Check sheet for the modelled part. Datum: model origin and axes. Units: mm. Face numbers are marked on the shaded views. A direction names the side the tool comes from. Give positions to 0.01 mm unless a question says otherwise; leave off trailing zeros. Order: outer loops, then holes, each group sorted by start corner. A loop starts at its lowest first (then second) coordinate and runs counter-clockwise, first axis right, second up.
```python
from build123d import *

# Parameters (mm, degrees)
F0_R     = 1.6
F1_DEPTH = 3.5
F3_COUNT = 16
F5_R     = 6.5
F6_DEPTH = 1
F7_R     = 6.5
F8_DEPTH = 1
F9_DEPTH = 12.5


with BuildPart() as f1:
    # F0 (on Top) → F1 (new body, symmetric)
    with BuildSketch(Plane.XY):
        with BuildLine():
            ThreePointArc((-0.6307960914, 4.7079290873), (-3.1277962342, -3.5748273689), (4.75, 0))
            ThreePointArc((4.75, 0), (3.5748273689, 3.1277962342), (0.6307960914, 4.7079290873))
            Line((0.6307960914, 4.7079290873), (0.75, 4.3804190402))
            Line((0.75, 4.3804190402), (-0.75, 4.3804190402))
            Line((-0.75, 4.3804190402), (-0.6307960914, 4.7079290873))
        make_face()
        Circle(F0_R, mode=Mode.SUBTRACT)
        with BuildLine():
            ThreePointArc((-0.6307960914, 4.7079290873), (0, 4.75), (0.6307960914, 4.7079290873))
            Line((0.6307960914, 4.7079290873), (0.3607043675, 5.45))
            Line((0.3607043675, 5.45), (-0.3607043675, 5.45))
            Line((-0.3607043675, 5.45), (-0.6307960914, 4.7079290873))
        make_face()
        with BuildLine():
            Line((0.75, 4.3804190402), (0.6307960914, 4.7079290873))
            ThreePointArc((0.6307960914, 4.7079290873), (0, 4.75), (-0.6307960914, 4.7079290873))
            Line((-0.6307960914, 4.7079290873), (-0.75, 4.3804190402))
            Line((-0.75, 4.3804190402), (0.75, 4.3804190402))
        make_face()
    extrude(amount=F1_DEPTH, both=True)


with BuildPart() as f3_1:
    # F3: instance of F1
    add(f1.part.rotate(Axis((0, 0, 0.113066053), (0, 0, -1)), 1 * 360 / F3_COUNT))


with BuildPart() as f3_2:
    # F3: instance of F1
    add(f1.part.rotate(Axis((0, 0, 0.113066053), (0, 0, -1)), 2 * 360 / F3_COUNT))


with BuildPart() as f3_3:
    # F3: instance of F1
    add(f1.part.rotate(Axis((0, 0, 0.113066053), (0, 0, -1)), 3 * 360 / F3_COUNT))


with BuildPart() as f3_4:
    # F3: instance of F1
    add(f1.part.rotate(Axis((0, 0, 0.113066053), (0, 0, -1)), 4 * 360 / F3_COUNT))


with BuildPart() as f3_5:
    # F3: instance of F1
    add(f1.part.rotate(Axis((0, 0, 0.113066053), (0, 0, -1)), 5 * 360 / F3_COUNT))


with BuildPart() as f3_6:
    # F3: instance of F1
    add(f1.part.rotate(Axis((0, 0, 0.113066053), (0, 0, -1)), 6 * 360 / F3_COUNT))


with BuildPart() as f3_7:
    # F3: instance of F1
    add(f1.part.rotate(Axis((0, 0, 0.113066053), (0, 0, -1)), 7 * 360 / F3_COUNT))


with BuildPart() as f3_8:
    # F3: instance of F1
    add(f1.part.rotate(Axis((0, 0, 0.113066053), (0, 0, -1)), 8 * 360 / F3_COUNT))


with BuildPart() as f3_9:
    # F3: instance of F1
    add(f1.part.rotate(Axis((0, 0, 0.113066053), (0, 0, -1)), 9 * 360 / F3_COUNT))


with BuildPart() as f3_10:
    # F3: instance of F1
    add(f1.part.rotate(Axis((0, 0, 0.113066053), (0, 0, -1)), 10 * 360 / F3_COUNT))


with BuildPart() as f3_11:
    # F3: instance of F1
    add(f1.part.rotate(Axis((0, 0, 0.113066053), (0, 0, -1)), 11 * 360 / F3_COUNT))


with BuildPart() as f3_12:
    # F3: instance of F1
    add(f1.part.rotate(Axis((0, 0, 0.113066053), (0, 0, -1)), 12 * 360 / F3_COUNT))


with BuildPart() as f3_13:
    # F3: instance of F1
    add(f1.part.rotate(Axis((0, 0, 0.113066053), (0, 0, -1)), 13 * 360 / F3_COUNT))


with BuildPart() as f3_14:
    # F3: instance of F1
    add(f1.part.rotate(Axis((0, 0, 0.113066053), (0, 0, -1)), 14 * 360 / F3_COUNT))


with BuildPart() as f3_15:
    # F3: instance of F1
    add(f1.part.rotate(Axis((0, 0, 0.113066053), (0, 0, -1)), 15 * 360 / F3_COUNT))


with BuildPart() as f3_1_1:
    add(f3_1.part)

    # F4: union F3_2, F3_3, F3_4, F3_5, F3_7, F3_9, F3_10, F3_8, F3_6, F3_11, F3_12, F3_14, F1, F3_13, F3_15
    add(f3_2.part)
    add(f3_3.part)
    add(f3_4.part)
    add(f3_5.part)
    add(f3_7.part)
    add(f3_9.part)
    add(f3_10.part)
    add(f3_8.part)
    add(f3_6.part)
    add(f3_11.part)
    add(f3_12.part)
    add(f3_14.part)
    add(f1.part)
    add(f3_13.part)
    add(f3_15.part)

    # F5 (on face) → F6 (join)
    with BuildSketch(Plane.XY.offset(3.5)):
        Circle(F5_R)
    extrude(amount=F6_DEPTH)

    # F7 (on face) → F8 (join)
    with BuildSketch(Plane(origin=(0, 0, -3.5), x_dir=(1, 0, 0), z_dir=(0, 0, -1))):
        Circle(F7_R)
    extrude(amount=F8_DEPTH)

    # F0 (on Top) → F9 (cut, symmetric)
    with BuildSketch(Plane.XY):
        Circle(F0_R)
    extrude(amount=F9_DEPTH, both=True, mode=Mode.SUBTRACT)


solid = f3_1_1.part
```
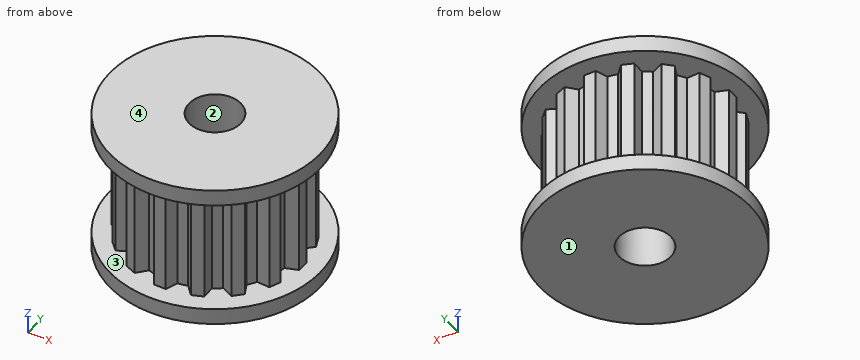
(1) Cross-section at A-A on x = 0. Enter the section's corners in (y, z).
Response values:
outline: (-6.5, -4.5) - (-1.6, -4.5) - (-1.6, 4.5) - (-6.5, 4.5) - (-6.5, 3.5) - (-5.45, 3.5) - (-5.45, -3.5) - (-6.5, -3.5) - close; (1.6, -4.5) - (6.5, -4.5) - (6.5, -3.5) - (5.45, -3.5) - (5.45, 3.5) - (6.5, 3.5) - (6.5, 4.5) - (1.6, 4.5) - close
(2) Gauge pin test, flat ends, axial feed: pin 1 Ø1 at (x, z) = (5, 0) entering from +Y; pin 2 Ø0.8 at (x, z) = (0, -1.5) entering from +Y; pin 3 Ø0.6 at (y, z) = (0, -1.5) entering from +X. Record the tip position at first contact, or that the pin passes through.
Response values:
pin 1: stops at y = 2.42
pin 2: stops at y = 5.45
pin 3: stops at x = 5.45
(3) Release check for a two-part mould opening along Y. For the marked faces 1 and 2 record: released by +Y, released by -Y, zero draft, split by the parting line, or undercut.
Response values:
face 1: zero draft
face 2: undercut
(4) Cross-section at C-C on x = -3.25. Enter the section's corners in (y, z), then the cut area to 3 significant figures.
Response values:
outline: (-5.63, -4.5) - (5.63, -4.5) - (5.63, -3.5) - (3.95, -3.5) - (3.95, 3.5) - (5.63, 3.5) - (5.63, 4.5) - (-5.63, 4.5) - (-5.63, 3.5) - (-3.95, 3.5) - (-3.95, -3.5) - (-5.63, -3.5) - close
area: 77.8 mm2
(5) Material ranges on L1, parallel to Z at x = 1.5, y = -5; L2, parallel to Y at x = 0, z = 1; L3, parallel to X at y = -5, z = 1.25, recorded low to high.
Response values:
L1: z = -4.5 to -3.5, 3.5 to 4.5
L2: y = -5.45 to -1.6, 1.6 to 5.45
L3: x = -2.17 to -1.59, -0.52 to 0.52, 1.59 to 2.17
(6) Set-up check for the marked faces 3 and 4: record each of +Z, -Z, +X, -X, +Y, -Y from which the full face is reachable in a straight line by a thin tool's end or side.
Response values:
face 3: none
face 4: +Z, +X, -X, +Y, -Y
